Verification items for the finished model (mm, model axes). A direction names the side the tool comes from. Give positions to 0.01 mm unless a question says otherwise; leave off trailing zeros. Write each loop counter-clockwise with the first axis right and the second up, starting at its lowest first coordinate (ties: lowest second). Pieces come first, ordered by that corner, then holes. Notation, with made-up numbers: (76.5, 5.5) -> (123.5, 5.5) arc R34 ccw to (123.5, 42.5) -> close; hole circle Ø4 at (68.25, -25). An arc over 180 degrees is marked (long way). Write item = value, one per line.
from build123d import *

# Parameters (mm, degrees)
EXTRUDE1_DEPTH     = 3.937
SKETCH2_R          = 2.794
CUT_EXTRUDE1_DEPTH = 0.254
SKETCH3_R          = 2.794
EXTRUDE2_DEPTH     = 0.635
SKETCH5_R          = 2.032
SKETCH5_R_2        = 1.778
EXTRUDE4_DEPTH     = 6.985
SKETCH6_R          = 2.794
SKETCH6_R_2        = 1.778
EXTRUDE5_DEPTH     = 0.254
EXTRUDE6_DEPTH     = 7.874
SKETCH8_R          = 2.54
CUT_EXTRUDE2_DEPTH = 3.556
SKETCH9_R          = 2.286
CUT_EXTRUDE3_DEPTH = 8.874
SKETCH10_R         = 3.175
CUT_EXTRUDE4_DEPTH = 0.635
CUT_EXTRUDE6_DEPTH = 3.048
SKETCH13_R         = 2.54
CUT_EXTRUDE7_DEPTH = 9.001
SKETCH14_R         = 3.175
CUT_EXTRUDE8_DEPTH = 0.635
EXTRUDE8_DEPTH     = 7.112


with BuildPart() as part:
    # Sketch1 → Extrude1 (new body)
    with BuildSketch(Plane(origin=(0, 0, 0), x_dir=(1, 0, 0), z_dir=(0, 1, 0))):
        with BuildLine():
            Line((-7.874, 3.937), (7.874, 3.937))
            ThreePointArc((7.874, 3.937), (11.811, 0), (7.874, -3.937))
            Line((7.874, -3.937), (-7.874, -3.937))
            ThreePointArc((-7.874, -3.937), (-11.811, 0), (-7.874, 3.937))
        make_face()
    extrude(amount=EXTRUDE1_DEPTH)

    # Sketch2 → Cut-Extrude1 (cut)
    with BuildSketch(Plane.XZ):
        Circle(SKETCH2_R)
    extrude(amount=-CUT_EXTRUDE1_DEPTH, mode=Mode.SUBTRACT)

    # Sketch3 → Extrude2 (add)
    with BuildSketch(Plane.XZ):
        with Locations((7.874, 0)):
            Circle(SKETCH3_R)
        with Locations((-7.874, 0)):
            Circle(SKETCH3_R)
    extrude(amount=EXTRUDE2_DEPTH)

    # Sketch5 → Extrude4 (add)
    with BuildSketch(Plane.XZ.offset(0.635)):
        with Locations((7.874, 0)):
            Circle(SKETCH5_R)
        with Locations((7.874, 0)):
            Circle(SKETCH5_R_2, mode=Mode.SUBTRACT)
        with Locations((-7.874, 0)):
            Circle(SKETCH5_R)
        with Locations((-7.874, 0)):
            Circle(SKETCH5_R_2, mode=Mode.SUBTRACT)
    extrude(amount=EXTRUDE4_DEPTH)

    # Sketch6 → Extrude5 (add)
    with BuildSketch(Plane.XZ.offset(7.62)):
        with Locations((-7.874, 0)):
            Circle(SKETCH6_R)
        with Locations((-7.874, 0)):
            Circle(SKETCH6_R_2, mode=Mode.SUBTRACT)
        with Locations((7.874, 0)):
            Circle(SKETCH6_R)
        with Locations((7.874, 0)):
            Circle(SKETCH6_R_2, mode=Mode.SUBTRACT)
    extrude(amount=-EXTRUDE5_DEPTH)

    # Sketch7 → Extrude6 (add)
    with BuildSketch(Plane(origin=(0, 0, -3.937), x_dir=(-1, 0, 0), z_dir=(0, 0, -1))):
        with BuildLine():
            Line((-7.874, 0), (7.874, 0))
            ThreePointArc((7.874, 0), (10.657879398, 1.153120602), (11.811, 3.937))
            Line((11.811, 3.937), (7.874, 3.937))
            Line((7.874, 3.937), (-7.874, 3.937))
            Line((-7.874, 3.937), (-11.811, 3.937))
            ThreePointArc((-11.811, 3.937), (-10.657879398, 1.153120602), (-7.874, 0))
        make_face()
    extrude(amount=-EXTRUDE6_DEPTH)

    # Sketch8 → Cut-Extrude2 (cut)
    with BuildSketch(Plane(origin=(0, 3.937, 0), x_dir=(1, 0, 0), z_dir=(0, 1, 0))):
        Circle(SKETCH8_R)
    extrude(amount=-CUT_EXTRUDE2_DEPTH, mode=Mode.SUBTRACT)

    # Sketch9 → Cut-Extrude3 (cut, through all)
    with BuildSketch(Plane.XY.offset(3.937)):
        with Locations((7.874, 3.937)):
            Circle(SKETCH9_R)
        with Locations((-7.874, 3.937)):
            Circle(SKETCH9_R)
    extrude(amount=-CUT_EXTRUDE3_DEPTH, mode=Mode.SUBTRACT)

    # Sketch10 → Cut-Extrude4 (cut)
    with BuildSketch(Plane.XY.offset(3.937)):
        with Locations((7.874, 3.937)):
            Circle(SKETCH10_R)
        with Locations((-7.874, 3.937)):
            Circle(SKETCH10_R)
    cut_extrude4 = extrude(amount=-CUT_EXTRUDE4_DEPTH, mode=Mode.SUBTRACT)

    # Mirror2: Cut-Extrude4 across plane
    add(cut_extrude4.mirror(Plane.XY), mode=Mode.SUBTRACT)

    # Sketch11 → Cut-Extrude6 (cut)
    with BuildSketch(Plane(origin=(0, 3.937, 0), x_dir=(1, 0, 0), z_dir=(0, 1, 0))):
        with BuildLine():
            Line((-5.08, -0.508), (-5.08, -2.794))
            Line((-5.08, -2.794), (-4.191, -2.794))
            Line((-4.191, -2.794), (-4.191, -3.937))
            Line((-4.191, -3.937), (4.191, -3.937))
            Line((4.191, -3.937), (4.191, -2.794))
            Line((4.191, -2.794), (5.08, -2.794))
            Line((5.08, -2.794), (5.08, -0.508))
            Line((5.08, -0.508), (3.00536853, -0.508))
            ThreePointArc((3.00536853, -0.508), (0, -3.048), (-3.00536853, -0.508))
            Line((-3.00536853, -0.508), (-5.08, -0.508))
        make_face()
        with BuildLine():
            Line((5.08, 0.508), (5.08, 2.794))
            Line((5.08, 2.794), (4.191, 2.794))
            Line((4.191, 2.794), (4.191, 3.937))
            Line((4.191, 3.937), (-4.191, 3.937))
            Line((-4.191, 3.937), (-4.191, 2.794))
            Line((-4.191, 2.794), (-5.08, 2.794))
            Line((-5.08, 2.794), (-5.08, 0.508))
            Line((-5.08, 0.508), (-3.00536853, 0.508))
            ThreePointArc((-3.00536853, 0.508), (0, 3.048), (3.00536853, 0.508))
            Line((3.00536853, 0.508), (5.08, 0.508))
        make_face()
    extrude(amount=-CUT_EXTRUDE6_DEPTH, mode=Mode.SUBTRACT)

    # Sketch13 → Cut-Extrude7 (cut, through all)
    with BuildSketch(Plane(origin=(0, 0.381, 0), x_dir=(1, 0, 0), z_dir=(0, 1, 0))):
        Circle(SKETCH13_R)
    extrude(amount=-CUT_EXTRUDE7_DEPTH, mode=Mode.SUBTRACT)

    # Sketch14 → Cut-Extrude8 (cut)
    with BuildSketch(Plane.XZ):
        Circle(SKETCH14_R)
    extrude(amount=-CUT_EXTRUDE8_DEPTH, mode=Mode.SUBTRACT)

    # Sketch17 → Extrude8 (add)
    with BuildSketch(Plane.XY.offset(3.937)):
        with BuildLine():
            Line((-4.064, 3.937), (-4.699, 3.937))
            ThreePointArc((-4.699, 3.937), (-7.874, 0.762), (-11.049, 3.937))
            Line((-11.049, 3.937), (-11.684, 3.937))
            ThreePointArc((-11.684, 3.937), (-7.874, 0.127), (-4.064, 3.937))
        make_face()
    extrude8 = extrude(amount=-EXTRUDE8_DEPTH)

    # Mirror3: Extrude8 across plane
    add(extrude8.mirror(Plane(origin=(0, 0, 0), x_dir=(0, 0, 1), z_dir=(1, 0, 0))))

    # Mirror1: part across face


with BuildPart() as part_1:
    add(part.part)
    add(part.part.mirror(Plane(origin=(0, 3.937, 0.023671087), x_dir=(0, 0, 1), z_dir=(0, 1, 0))))


solid = part_1.part
Item 1: Sectioned sample at C-C on z = -1. Give the number of separate pieces and of enclosed holes in the cut face, then the cut area to 3 significant figures.
Response values:
separate_pieces = 2
enclosed_holes = 6
area = 123 mm^2
Item 2: Sectioned sample at B-B on y = -5. Record the cut outline in (x, z).
Response values:
outline = circle Ø4.06 at (-7.87, 0); circle Ø4.06 at (7.87, 0); hole circle Ø3.56 at (-7.87, 0); hole circle Ø3.56 at (7.87, 0)
Item 3: Go/stop test with flat-tipped pins: P1, Ø1.8, axis at x = -8.5, z = 0, coming from the +Y side; P2, Ø4, axis at x = 7.874, z = 0, coming from the -Y side; P3, Ø3, axis at x = 7.874, z = 0, coming from the -Y side (3 decimals); P4, Ø4, axis at y = -3.5, z = -1.5, coming from the -X side. Record where each tip stops, or that it passes through.
Response values:
P1 = 8.51
P2 = -7.62
P3 = -0.635
P4 = -9.91
Item 4: Sectioned sample at A-A on x = 0. Record the cut outline in (y, z) (3 decimals), then the cut area to 3 significant figures.
Response values:
outline = (0, -3.937) -> (0.889, -3.937) -> (0.889, -3.048) -> (6.985, -3.048) -> (6.985, -3.937) -> (7.874, -3.937) -> (7.874, -3.175) -> (7.239, -3.175) -> (7.239, -2.54) -> (0.635, -2.54) -> (0.635, -3.175) -> (0, -3.175) -> close; (0, 3.175) -> (0.635, 3.175) -> (0.635, 2.54) -> (7.239, 2.54) -> (7.239, 3.175) -> (7.874, 3.175) -> (7.874, 3.937) -> (6.985, 3.937) -> (6.985, 3.048) -> (0.889, 3.048) -> (0.889, 3.937) -> (0, 3.937) -> close
area = 9.55 mm^2
Item 5: Set-up check for faces 1 (the cylindrical face through (-4.846, 4.891, -3.624)), 2 (the flat face through (-8, 8.509, 0)), 3 (the flat face through (7, -0.635, -2)): record each of +Z, -Z, +X, -X, +Y, -Y from which the full face is reachable in a straight line by a thin tool's end or side.
Response values:
face_1 = -Z
face_2 = +Y
face_3 = none
Item 6: Material ranges on line 1 (Y direction, x = -1, z = -3.5) (3 decimals); line 2 (X direction, y = 2.25, z = 1); line 3 (X direction, y = 11.5, z = -1.5), recorded low to high.
Response values:
line_1 = 0 to 0.889, 6.985 to 7.874
line_2 = -11.68 to -9.42, -6.33 to -4.46, -2.88 to -2.33, 2.33 to 2.88, 4.46 to 6.33, 9.42 to 11.68
line_3 = -9.24 to -8.83, -6.92 to -6.5, 6.5 to 6.92, 8.83 to 9.24
